Check sheet for the modelled part. Datum: model origin and axes. Units: mm. Coordinates: 2 decimals unless noted, no trailing zeros. Write each loop counter-clockwise with the first axis right and the second up, starting at its lowest first coordinate (ties: lowest second). Pieces come first, ordered by that corner, then holes. Notation, with made-up numbers: M 55.5,46 L 103.5,46 A11 ccw 103.5,67 Z; hole C 36.5,58 d4. An arc over 180 degrees is marked long. Answer as CSV lines item,"result". Start each with the question number.
Q1. Depth check by flat-ended pin: pin 1 Ø1.5 at (y, z) = (-177.5, 4.5) entering from +X; pin 2 Ø16 at (x, y) = (-25, -25) entering from +Z; pin 3 Ø1.5 at (x, z) = (142.5, 3) entering from -Y; pin 4 Ø1 at (y, z) = (-171, 1.5) entering from -X. Enter the tip coordinate at first touch or a pass-through.
Q2. Thickness scan on line 1 along Y through (x, z) = (25, 3.95); line 2 along Y through (x, z) = (-74, 1.25); line 3 along X through (y, z) = (-119.5, 2.2). Record the ranges inside material, lowest first. Write a range as from..to.
Q3. Sectioned sample at C-C, the plane x = 25. Record the cut outline in (y, z), then the cut area to 3 significant figures.
Q4. Sectioned sample at A-A, the plane y = -25. Record the cut outline in (x, z), then the cut area to 3 significant figures.
Q5. Sectioned sample at B-B, the plane x = 125. Record the cut outline in (y, z), then the cut area to 3 significant figures.
Q6. Sectioned sample at D-D, the plane y = -171. Record the cut outline in (x, z).
from build123d import *

# Parameters (mm, degrees)
F1_DEPTH = 5
F2_R     = 9
F3_DEPTH = 25
F4_R     = 10


with BuildPart() as f1:
    # F0 (on Top) → F1 (new body)
    with BuildSketch(Plane.XY):
        Polygon((200, 0), (0, 0), (-200, 0), (-200, -100), (-100, -100), (-100, -200), (0, -200), (100, -200), (100, -100), (200, -100), align=None)
    extrude(amount=F1_DEPTH)

    # F2 (on face) → F3 (cut)
    with BuildSketch(Plane.XY.offset(5)):
        with Locations((175.068656, -74.99178)):
            Circle(F2_R)
        with Locations((125, -25)):
            Circle(F2_R)
        with Locations((75.068656, -74.99178)):
            Circle(F2_R)
        with Locations((75.068656, -174.99178)):
            Circle(F2_R)
        with Locations((25.068656, -124.99178)):
            Circle(F2_R)
        with Locations((25, -25)):
            Circle(F2_R)
        with Locations((-75.068656, -174.99178)):
            Circle(F2_R)
        with Locations((-25, -25)):
            Circle(F2_R)
        with Locations((-175.068656, -74.99178)):
            Circle(F2_R)
        with Locations((-125, -25)):
            Circle(F2_R)
        with Locations((-75.068656, -74.99178)):
            Circle(F2_R)
        with Locations((-25.068656, -124.99178)):
            Circle(F2_R)
    extrude(amount=-F3_DEPTH, mode=Mode.SUBTRACT)

    # F4
    f4_edges = [f1.edges().sort_by_distance(p)[0] for p in [
        (-100, -200, 2.5),
        (100, -200, 2.5),
        (200, -100, 2.5),
        (200, 0, 2.5),
        (-200, -100, 2.5),
        (-200, 0, 2.5),
    ]]
    fillet(f4_edges, radius=F4_R)


solid = f1.part
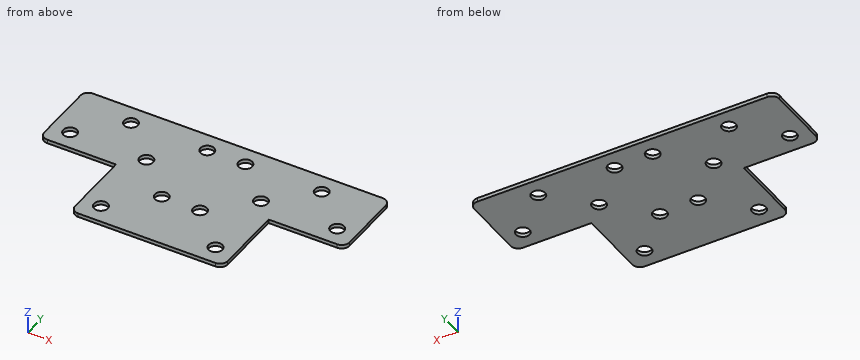
Output:
1,pin 1,"stops at x = 100"
1,pin 2,"passes through"
1,pin 3,"stops at y = -100"
1,pin 4,"stops at x = -100"
2,line 1,"y = -200..-133.99, -115.99..-34, -16..0"
2,line 2,"y = -200..-183.93, -166.06..-83.93, -66.06..0"
2,line 3,"x = -100..-32.2, -17.94..17.94, 32.2..100"
3,outline,"M -200,0 L -133.99,0 L -133.99,5 L -200,5 Z; M -115.99,0 L -34,0 L -34,5 L -115.99,5 Z; M -16,0 L 0,0 L 0,5 L -16,5 Z"
3,area,"820 mm^2"
4,outline,"M -200,0 L -134,0 L -134,5 L -200,5 Z; M -116,0 L -34,0 L -34,5 L -116,5 Z; M -16,0 L 16,0 L 16,5 L -16,5 Z; M 34,0 L 116,0 L 116,5 L 34,5 Z; M 134,0 L 200,0 L 200,5 L 134,5 Z"
4,area,"1,640 mm^2"
5,outline,"M -100,0 L -34,0 L -34,5 L -100,5 Z; M -16,0 L 0,0 L 0,5 L -16,5 Z"
5,area,"410 mm^2"
6,outline,"M -100,0 L -83.13,0 L -83.13,5 L -100,5 Z; M -67,0 L 67,0 L 67,5 L -67,5 Z; M 83.13,0 L 100,0 L 100,5 L 83.13,5 Z"
